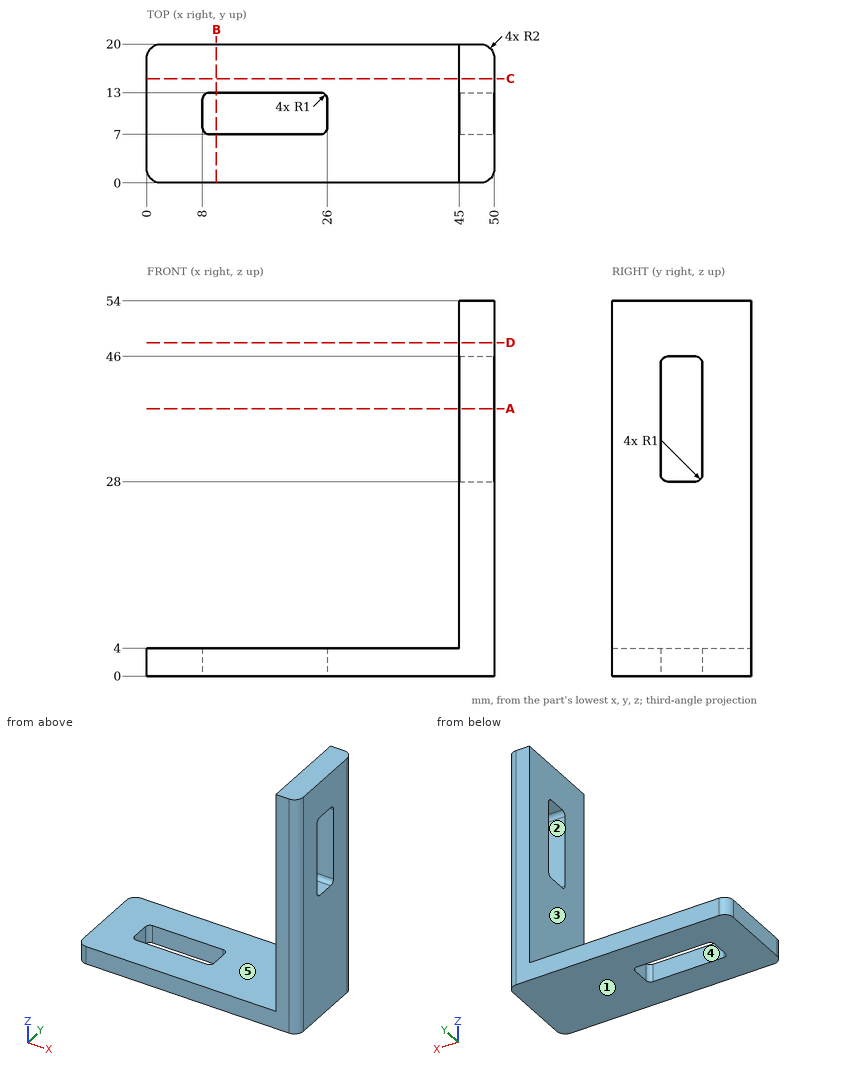
Study the drawing (mm; zero at the part's minimum x, y, z) and answer. A direction names the side the tool comes from. Give positions to 0.01 mm unless a question says otherwise; leave off trailing zeros. Write each loop counter-clockwise with the first axis right and the second up, starting at its lowest first coordinate (ties: lowest second). Pieces come first, ordered by that corner, then holes. Notation, with made-up numbers: (83, 63.5) -> (125, 63.5) arc R23 ccw to (125, 78.5) -> close; hole circle Ø6 at (7.5, 5). An arc over 180 degrees is marked (long way). Write item = value, one per line. Start each with the question number.
1) The part is cut by section C-C, the plane y = 15. Determine the outline of the cut face in (x, z).
2) Determine the mould class of the marked faces 3, 4 and 5 for opening direction X: +X half, -X half, draft (parallel to the pull), parting line (faces both ways), or undercut.
3) The part is cut by section B-B, the plane x = 10. Determine the outline of the cut face in (y, z).
4) Straight lines are drawn through the part: line 1 along X through (y, z) = (18.25, 45); line 2 along Z through (x, y) = (12, 5); line 3 along X through (y, z) = (12.75, 3.5). For each, find the intervals that lie inside material, in ascending order.
5) The part is cut by section A-A, the plane z = 38.5. Determine the outline of the cut face in (x, y), and give its area (3 significant figures).
6) Which of the six approach directions +Z, -Z, +X, -X, +Y, -Y give full straight-line access (tool end or side, diameter ignored) to the marked faces 1 and 2?
7) Each of these flat-tipped pins is pushed along its axis until it touches: pin 1 (6 mm diameter, centred on y = 12, z = 29.5, fed in from -X); pin 2 (5 mm diameter, centred on x = 13, y = 4.5, fed in from +Z); pin 3 (2 mm diameter, centred on x = 43, z = 37, fed in from +Y). Where does it stop, or does it pass through?
8) The part is cut by section D-D, the plane z = 48. Determine the outline of the cut face in (x, y), and give its area (3 significant figures).
Solutions:
q1.outline = (0, 0) -> (50, 0) -> (50, 54) -> (45, 54) -> (45, 4) -> (0, 4) -> close
q2.face_3 = -X half
q2.face_4 = undercut
q2.face_5 = draft
q3.outline = (0, 0) -> (7, 0) -> (7, 4) -> (0, 4) -> close; (13, 0) -> (20, 0) -> (20, 4) -> (13, 4) -> close
q4.line_1 = 45 to 49.98
q4.line_2 = 0 to 4
q4.line_3 = 0 to 8.34, 25.66 to 50
q5.outline = (45, 0) -> (48, 0) arc R2 ccw to (50, 2) -> (50, 7) -> (45, 7) -> close; (45, 13) -> (50, 13) -> (50, 18) arc R2 ccw to (48, 20) -> (45, 20) -> close
q5.area = 68.3 mm²
q6.face_1 = -Z, +X, -X, +Y, -Y
q6.face_2 = +X, -X
q7.pin_1 = 45
q7.pin_2 = 4
q7.pin_3 = through
q8.outline = (45, 0) -> (48, 0) arc R2 ccw to (50, 2) -> (50, 18) arc R2 ccw to (48, 20) -> (45, 20) -> close
q8.area = 98.3 mm²
